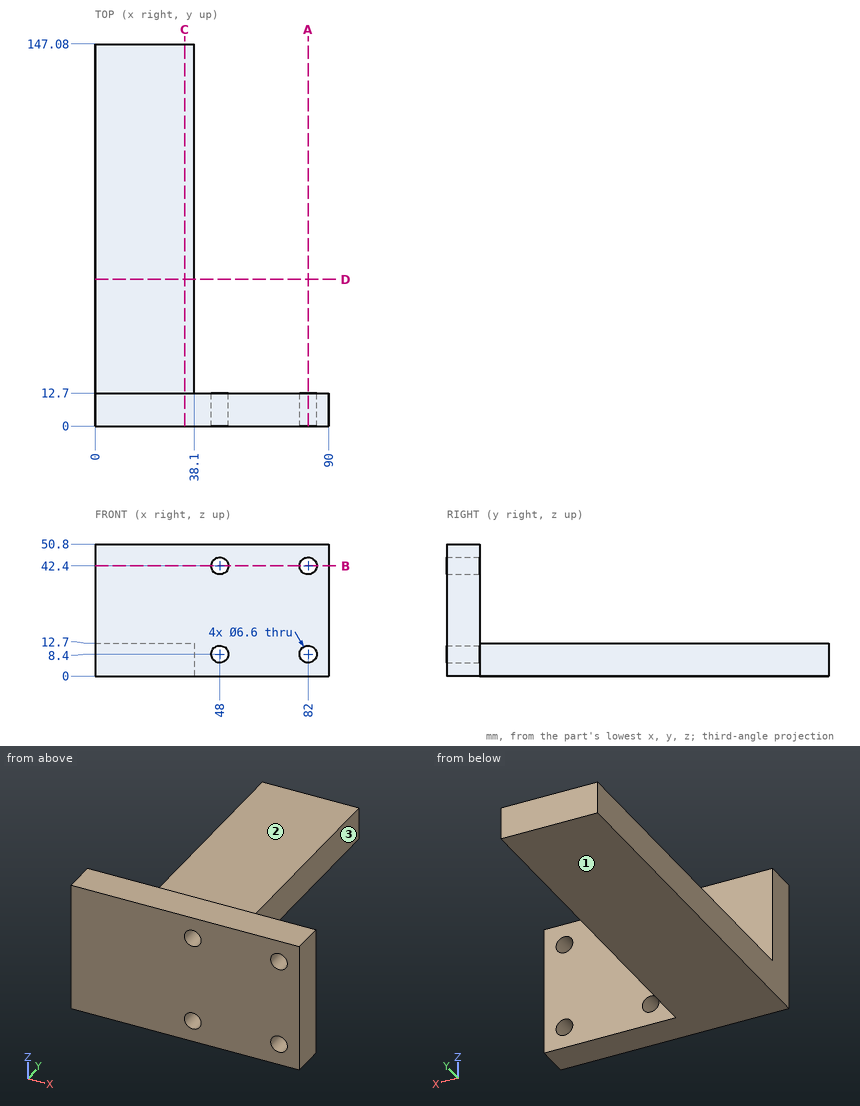
Geometry: see drawing. Coordinates: mm, zero at the bounding-box minimum. A direction names the side the tool comes from. Round coordinates to 2 decimals unless told otherwise and drop trailing zeros. Loops run counter-clockwise (first coordinate to the right, second up) from the corner with the lowest first, then second, coordinate; pieces in that order, holes last. Notation, with made-up numbers: (42.25, 12.25) -> (98.25, 12.25) arc R19 ccw to (98.25, 20.25) -> close; hole circle Ø6 at (-6, -8). An arc over 180 degrees is marked (long way). Write each question's results on one line, items separated by ' | '.
Item 1: Cut plane A-A on x = 82. Return the cut outline in (y, z).
Answers below:
outline: (0, 0) -> (12.7, 0) -> (12.7, 5.1) -> (0, 5.1) -> close; (0, 11.7) -> (12.7, 11.7) -> (12.7, 39.1) -> (0, 39.1) -> close; (0, 45.7) -> (12.7, 45.7) -> (12.7, 50.8) -> (0, 50.8) -> close
Item 2: Cut plane D-D on y = 56.5. Return the cut outline in (x, z).
Answers below:
outline: (0, 0) -> (38.1, 0) -> (38.1, 12.7) -> (0, 12.7) -> close
Item 3: Line query: probe 1 along X at (y, z) = (3.25, 42.4); probe 2 along Z at (x, y) = (48, 6); probe 3 along X at (y, z) = (81.5, 11). Output: solid intervals per line, ascending. Write a range as [from, to].
Answers below:
probe 1: x = [0, 44.7], [51.3, 78.7], [85.3, 90] | probe 2: z = [0, 5.1], [11.7, 39.1], [45.7, 50.8] | probe 3: x = [0, 38.1]
Item 4: Cut plane C-C on x = 34.5. Return the cut outline in (y, z), and give its area (3 significant figures).
Answers below:
outline: (0, 0) -> (147.08, 0) -> (147.08, 12.7) -> (12.7, 12.7) -> (12.7, 50.8) -> (0, 50.8) -> close | area: 2,350 mm²
Item 5: Cut plane B-B on z = 42.4. Return the cut outline in (x, y).
Answers below:
outline: (0, 0) -> (44.7, 0) -> (44.7, 12.7) -> (0, 12.7) -> close; (51.3, 0) -> (78.7, 0) -> (78.7, 12.7) -> (51.3, 12.7) -> close; (85.3, 0) -> (90, 0) -> (90, 12.7) -> (85.3, 12.7) -> close
Item 6: Pin query (flat end, axial travel): pin 1 Ø8 at (x, z) = (72.5, 7.5) entering from +Y; pin 2 Ø14 at (y, z) = (54.5, 4.5) entering from +X; pin 3 Ø11.5 at (x, y) = (15.5, 69) entering from +Z. Return the tip coordinate at first contact, or that it passes through.
Answers below:
pin 1: stops at y = 12.7 | pin 2: stops at x = 38.1 | pin 3: stops at z = 12.7
Item 7: Set-up query: the marked faces 1, 2 and 3. Return all of +Z, -Z, +X, -X, +Y, -Y with unobstructed straight access to the full face (end or side cutting, diameter ignored); none if empty.
Answers below:
face 1: -Z, +X, -X, +Y, -Y | face 2: +Z, +X, -X, +Y | face 3: +Z, -Z, +X, +Y
